```python
from build123d import *

# Parameters (mm, degrees)
SKETCH1_R           = 43.815
SKETCH1_R_2         = 41.275
EXTRUDE_THIN1_DEPTH = 50.8
BOSS_EXTRUDE1_START = 2.54
BOSS_EXTRUDE1_DEPTH = 2.54


with BuildPart() as part:
    # Sketch1 → Extrude-Thin1 (new body)
    with BuildSketch(Plane(origin=(0, 0, 0), x_dir=(1, 0, 0), z_dir=(0, 1, 0))):
        Circle(SKETCH1_R)
        Circle(SKETCH1_R_2, mode=Mode.SUBTRACT)
    extrude(amount=EXTRUDE_THIN1_DEPTH)

    # Sketch2 → Boss-Extrude1 (add)
    with BuildSketch(Plane.XZ.offset(BOSS_EXTRUDE1_START)):
        with BuildLine():
            Line((0, -43.815), (0, 0))
            Line((0, 0), (-37.944903067, -21.9075))
            ThreePointArc((-37.944903067, -21.9075), (21.9075, 37.944903067), (0, -43.815))
        make_face()
    extrude(amount=-BOSS_EXTRUDE1_DEPTH)


solid = part.part
```
Design review of the part built by this model. Coordinates are the model's own, in mm. A direction names the side the tool comes from. Coordinates: 2 decimals unless noted, no trailing zeros. Loops run counter-clockwise (first coordinate to the right, second up) from the corner with the lowest first, then second, coordinate; pieces in that order, holes last.
Q1. We need section B-B on x = -10.5. State the section outline as (y, z) points, and give its area (3 significant figures).
Reported:
outline: (-2.54, -6.06) - (0, -6.06) - (0, 39.92) - (50.8, 39.92) - (50.8, 42.54) - (-2.54, 42.54) - close; (0, -42.54) - (50.8, -42.54) - (50.8, -39.92) - (0, -39.92) - close
area: 390 mm2
Q2. For pin 1 (1.5 mm diameter, centred on x = 20, y = 19.5, fed in from +Z); pin 2 (1.3 mm diameter, centred on y = -1.5, z = -30.5, fed in from -X); pin 3 (5 mm diameter, centred on x = 25, y = 44, fed in from +Z), all flat-tipped, find the tip position at first contact; note any pin that passes through.
Reported:
pin 1: stops at z = 39.36
pin 2: stops at x = 0
pin 3: stops at z = 37.6
Q3. We need section C-C on y = 35.5. State the section outline as (x, z) points (3 decimals), and give its area (3 significant figures).
Reported:
outline: circle Ø87.63 at (0, 0); hole circle Ø82.55 at (0, 0)
area: 679 mm2
Q4. We need section A-A on z = -15. State the section outline as (x, y) points.
Reported:
outline: (-41.17, -2.54) - (-25.98, -2.54) - (-25.98, 0) - (-38.45, 0) - (-38.45, 50.8) - (-41.17, 50.8) - close; (0, -2.54) - (41.17, -2.54) - (41.17, 50.8) - (38.45, 50.8) - (38.45, 0) - (0, 0) - close
Q5. Tool access review of faces 3 (the face through (1, -2.54, 1)), 4 (the face through (-8.948, 25.044, 40.293)): name each direction out of +Z, -Z, +X, -X, +Y, -Y from which nothing blocks a thin tool from reaching the whole face with its end or side.
Reported:
face 3: +Z, -Z, +X, -X, -Y
face 4: +Y
Q6. The part is to be moulded in two halves that separate along X. For faces 1 (the face through (16, 50.8, 39)), 2 (the face through (0, -1, -22)), say which applies: +X half, -X half, draft (parallel to the pull), parting line (faces both ways), or undercut.
Reported:
face 1: draft
face 2: undercut
Q7. To check wall thickness, follow line 1 (X direction, y = 32.5, z = 0) (3 decimals); line 2 (Z direction, x = 29, y = 9). State the ranges of each line that lie inside material, in increasing order.
Reported:
line 1: x = -43.815 to -41.275, 41.275 to 43.815
line 2: z = -32.84 to -29.37, 29.37 to 32.84
Q8. We need section D-D on z = 6.5. State the section outline as (x, y) points.
Reported:
outline: (-43.33, -2.54) - (43.33, -2.54) - (43.33, 50.8) - (40.76, 50.8) - (40.76, 0) - (-40.76, 0) - (-40.76, 50.8) - (-43.33, 50.8) - close
